Design review of the part built by this model. Coordinates are the model's own, in mm. Face numbers are marked on the shaded views. A direction names the side the tool comes from. Give positions to 0.01 mm unless a question says otherwise; leave off trailing zeros. Loops run counter-clockwise (first coordinate to the right, second up) from the corner with the lowest first, then second, coordinate; pieces in that order, holes last. Notation, with made-up numbers: (34.25, -11.75) - (77.25, -11.75) arc R22 ccw to (77.25, 25.25) - close; hole circle Ø3 at (54, -16.5). An arc over 180 degrees is marked (long way). One line per item, written item: value. Start each with the question number.
```python
from build123d import *

# Parameters (mm, degrees)
SKETCH1_R           = 7.5
BOSS_EXTRUDE1_DEPTH = 28
CUT_EXTRUDE1_DEPTH  = 30.941609843
CIRPATTERN1_COUNT   = 5


with BuildPart() as part:
    # Sketch1 → Boss-Extrude1 (new body)
    with BuildSketch(Plane.XY):
        Circle(SKETCH1_R)
    extrude(amount=BOSS_EXTRUDE1_DEPTH)

    # Sketch2 → Cut-Extrude1 (cut, through all)
    with BuildSketch(Plane.XY):
        Polygon((0, 3.429306859), (-1.35645876, 4.852854397), (-4.219139018, 6.200714954), (0, 11.25164702), (4.219139018, 6.200714954), (1.35645876, 4.852854397), align=None)
    cut_extrude1 = extrude(amount=CUT_EXTRUDE1_DEPTH, mode=Mode.SUBTRACT)

    # CirPattern1: Cut-Extrude1 ×5 about axis
    cirpattern1_axis = Axis((0, 0, 0), (0, 0, 1))
    for i in range(1, CIRPATTERN1_COUNT):
        add(cut_extrude1.rotate(cirpattern1_axis, i * 360 / CIRPATTERN1_COUNT), mode=Mode.SUBTRACT)


solid = part.part
```
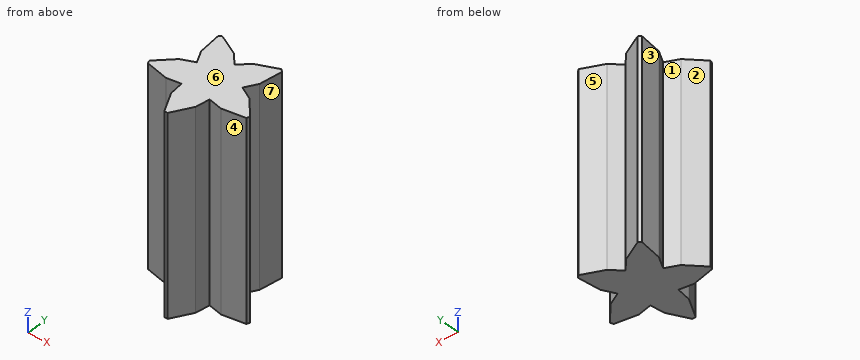
(1) Take a section at A-A on z = 14. State the section outline as (x, y) points, and give its area (3 significant figures).
(2) Draft analysis for pull direction Y (two halves, no side actions). For the marked faces 1, 2, 3 and 4, state which applies: pulls with the +Y half, pulls with the -Y half, needs draft (parallel to the pull), parting line crosses it, or undercut.
(3) For pin 1 Ø1 at (x, z) = (0, 18.5) entering from +Y; pin 2 Ø8 at (x, z) = (-5.5, 4.5) entering from -Y; pin 3 Ø2 at (y, z) = (4, 14.5) entering from -X, all flat-tipped, find the tip position at first contact; note any pin that passes through.
(4) To check wall thickness, follow L1, parallel to X at y = 4, z = 10.5; L2, parallel to Y at x = -3.5, z = 9.25; L3, parallel to X at y = -5, z = 1.5. State the ranges of each line that lie inside material, in increasing order. Write a range as from..to.
(5) Take a section at C-C on x = -0.75. State the section outline as (y, z) points, and give its area (3 significant figures).
(6) Machinability: for the marked faces 5, 6 and 7, which of the approach directions +Z, -Z, +X, -X, +Y, -Y give a long, thin tool a straight path to every point of the face, cutting with its end or side? Answer none if there is none.
(7) Take a section at B-B on y = -5. State the section outline as (x, z) points, and give its area (3 significant figures).
Here are the results:
1. outline: (-7.2, -2.1) arc R7.5 ccw to (-7.06, -2.54) - (-3.95, -3.13) - (-2.02, -2.77) - (-1.76, -4.72) - (-0.23, -7.5) arc R7.5 ccw to (0.23, -7.5) - (1.76, -4.72) - (2.02, -2.77) - (3.95, -3.13) - (7.06, -2.54) arc R7.5 ccw to (7.2, -2.1) - (5.03, 0.21) - (3.26, 1.06) - (4.2, 2.79) - (4.59, 5.93) arc R7.5 ccw to (4.22, 6.2) - (1.36, 4.85) - (0, 3.43) - (-1.36, 4.85) - (-4.22, 6.2) arc R7.5 ccw to (-4.59, 5.93) - (-4.2, 2.79) - (-3.26, 1.06) - (-5.03, 0.21) - close
1. area: 92.3 mm²
2. face 1: undercut
2. face 2: pulls with the +Y half
2. face 3: undercut
2. face 4: pulls with the -Y half
3. pin 1: y = 3.95
3. pin 2: y = -5.19
3. pin 3: x = -4.48
4. L1: -4.35..-0.54, 0.54..4.35
4. L2: -3.05..0.95, 1.5..5.86
4. L3: -1.6..1.6
5. outline: (-6.55, 0) - (4.22, 0) - (4.22, 28) - (-6.55, 28) - close
5. area: 302 mm²
6. face 5: +Z, -Z, +Y
6. face 6: +Z, +X, -X, +Y, -Y
6. face 7: +Z, -Z, +X
7. outline: (-1.6, 0) - (1.6, 0) - (1.6, 28) - (-1.6, 28) - close
7. area: 89.8 mm²
